```python
from build123d import *

# Parameters (mm, degrees)
PAD_DEPTH         = 1.5
CYLINDER001_R     = 2.2
CYLINDER001_DEPTH = 10
CYLINDER_R        = 4.4
CYLINDER_DEPTH    = 10
BOX001_W          = 3
BOX001_H          = 18
BOX001_DEPTH      = 20
FILLET001_R       = 3
BOX_W             = 20
BOX_H             = 18
BOX_DEPTH         = 6
FILLET_R          = 2


with BuildPart() as side_wall_body:
    # Sketch → Pad (new body)
    with BuildSketch(Plane.XZ):
        with BuildLine():
            Line((0, 11.694638), (0, 0))
            Line((0, 0), (14.6909, 0))
            add(Edge.make_bspline(
                [(0, 11.694638), (7.772997, 9.987508), (9.324936, 7.918261), (11.342452, 6.262862), (12.842653, 5.228237), (14.084202, 4.193611), (15.118829, 2.176094), (14.6909, 0)],
                knots=[0, 0, 0, 0, 0.2, 0.4, 0.6, 0.8, 1, 1, 1, 1], degree=3))
        make_face()
    extrude(amount=PAD_DEPTH)


with BuildPart() as side_wall_fusion:
    # Part__Mirroring: instance of side wall body
    add(side_wall_body.part.mirror(Plane(origin=(0, 7.5, 0), x_dir=(1, 0, 0), z_dir=(0, 1, 0))))

    # Fusion002: union side wall body
    add(side_wall_body.part)


with BuildPart() as side_wall_fusion_1:
    # Fusion002 placement: moved
    add(side_wall_fusion.part.moved(Location((0, 1.5, 0))))


with BuildPart() as bolt_hole:
    # Cylinder001 → Cylinder001 (new body)
    with BuildSketch(Plane(origin=(15, 9, -4), x_dir=(1, 0, 0), z_dir=(0, 0, 1))):
        Circle(CYLINDER001_R)
    extrude(amount=CYLINDER001_DEPTH)


with BuildPart() as hole_fusion:
    # Cylinder → Cylinder (new body)
    with BuildSketch(Plane(origin=(-3, 9, 19.6), x_dir=(0, 0, -1), z_dir=(1, 0, 0))):
        Circle(CYLINDER_R)
    extrude(amount=CYLINDER_DEPTH)

    # Fusion001: union bolt hole
    add(bolt_hole.part)


with BuildPart() as socket_fillet:
    # Box001 → Box001 (new body)
    with BuildSketch(Plane.XY.offset(6)):
        with Locations((1.5, 9)):
            Rectangle(BOX001_W, BOX001_H)
    extrude(amount=BOX001_DEPTH)

    # Fillet001
    fillet001_edges = [socket_fillet.edges().sort_by_distance(p)[0] for p in [
        (1.5, 0, 26),
        (1.5, 18, 26),
    ]]
    fillet(fillet001_edges, radius=FILLET001_R)


with BuildPart() as power_12v_socket_fusion:
    # Box → Box (new body)
    with BuildSketch(Plane.XY):
        with Locations((10, 9)):
            Rectangle(BOX_W, BOX_H)
    extrude(amount=BOX_DEPTH)

    # Fillet
    fillet_edges = [power_12v_socket_fusion.edges().sort_by_distance(p)[0] for p in [
        (20, 0, 3),
        (20, 18, 3),
    ]]
    fillet(fillet_edges, radius=FILLET_R)

    # Fusion: union socket fillet
    add(socket_fillet.part)

    # Cut: cut hole fusion
    add(hole_fusion.part, mode=Mode.SUBTRACT)

    # Fusion003: union side wall fusion
    add(side_wall_fusion_1.part)


solid = power_12v_socket_fusion.part
```
Source: CAD feature listing. Evaluate the final solid. Frame: model axes, mm. A direction names the side the tool comes from. Round coordinates to 2 decimals unless told otherwise and drop trailing zeros. Order: outer loops, then holes, each group sorted by start corner. A loop starts at its lowest first (then second) coordinate and runs counter-clockwise, first axis right, second up. Notation, with made-up numbers: (21, 38) -> (57, 38) arc R18 ccw to (57, 46) -> close; hole circle Ø3 at (50, 55). An arc over 180 degrees is marked (long way). Use CSV: the item, a comma, the result in double quotes.
(1) Ray query, L1, parallel to X at y = 9, z = 1.7; L2, parallel to Y at x = 2.3, z = 19.6; L3, parallel to Y at x = 15, z = 1.3. Return the intervals inside material, ascending.
Report:
L1,"0 to 12.8, 17.2 to 20"
L2,"0 to 4.6, 13.4 to 18"
L3,"0 to 6.8, 11.2 to 18"
(2) First-contact query: pin 1 Ø2 at (x, y) = (6.5, 15) entering from +Z; pin 2 Ø9 at (y, z) = (10.5, 16.5) entering from +X; pin 3 Ø2 at (x, z) = (6.5, 12.5) entering from -Y. Flat tips, straight axial feed; report the tip coordinate or a pass-through.
Report:
pin 1,"z = 6"
pin 2,"x = 3"
pin 3,"through"
(3) Section D-D on x = 1.75. Return the cut outline in (y, z), and give its area (3 significant figures).
Report:
outline,"(0, 0) -> (18, 0) -> (18, 23) arc R3 ccw to (15, 26) -> (3, 26) arc R3 ccw to (0, 23) -> close; hole circle Ø8.8 at (9, 19.6)"
area,"403 mm^2"
(4) Section A-A on x = 15. Return the cut outline in (y, z), and give its area (3 significant figures).
Report:
outline,"(0, 0) -> (6.8, 0) -> (6.8, 6) -> (0, 6) -> close; (11.2, 0) -> (18, 0) -> (18, 6) -> (11.2, 6) -> close"
area,"81.6 mm^2"
(5) Access query for faces 4 (the face through (1, 9, 26)), 5 (the face through (6, 1.5, 8)). Directions: +Z, -Z, +X, -X, +Y, -Y. A direction counts if a zero-diameter tool reaches every point of the face in a straight line with its end or side. Return the directions, or none.
Report:
face 4,"+Z, +X, -X, +Y, -Y"
face 5,"+Z, +X"
(6) Pull-direction query (Z, two-part tool) for faces 1 (the face through (1.479, 10.322, 15.403)), 2 (the face through (7, 18, 6)), 3 (the face through (1.52, 17.14, 25.1)); classes: +Z half, -Z half, draft (parallel to the pull), parting line (faces both ways), or undercut.
Report:
face 1,"undercut"
face 2,"draft"
face 3,"+Z half"
(7) Section C-C on z = 19.6. Return the cut outline in (x, y).
Report:
outline,"(0, 0) -> (3, 0) -> (3, 4.6) -> (0, 4.6) -> close; (0, 13.4) -> (3, 13.4) -> (3, 18) -> (0, 18) -> close"
(8) Section B-B on y = 9. Return the cut outline in (x, z), and give its area (3 significant figures).
Report:
outline,"(0, 0) -> (12.8, 0) -> (12.8, 6) -> (3, 6) -> (3, 15.2) -> (0, 15.2) -> close; (0, 24) -> (3, 24) -> (3, 26) -> (0, 26) -> close; (17.2, 0) -> (20, 0) -> (20, 6) -> (17.2, 6) -> close"
area,"127 mm^2"
